Design review of the part built by this model. Coordinates are the model's own, in mm. Coordinates: 2 decimals unless noted, no trailing zeros. Loops run counter-clockwise (first coordinate to the right, second up) from the corner with the lowest first, then second, coordinate; pieces in that order, holes last. Notation, with made-up numbers: (56.25, 19.25) - (72.25, 19.25) arc R10 cw to (72.25, 36.25) - close; hole circle Ø9 at (-33, 53). An arc over 180 degrees is marked (long way). One line per question, with ' | ' between items.
from build123d import *

# Parameters (mm, degrees)
SKETCH1_W           = 10
SKETCH1_H           = 5
BOSS_EXTRUDE1_DEPTH = 0.6
SKETCH2_W           = 1.15
SKETCH2_H           = 2.7
CUT_EXTRUDE1_DEPTH  = 6.622277119
SKETCH3_R           = 0.15
CUT_EXTRUDE2_DEPTH  = 6.622277119


with BuildPart() as part:
    # Sketch1 → Boss-Extrude1 (new body)
    with BuildSketch(Plane.XY):
        Rectangle(SKETCH1_W, SKETCH1_H)
    extrude(amount=BOSS_EXTRUDE1_DEPTH)

    # Sketch2 → Cut-Extrude1 (cut, through all)
    with BuildSketch(Plane.XY.offset(0.6)):
        with Locations((-4.425, -1.15)):
            Rectangle(SKETCH2_W, SKETCH2_H)
    extrude(amount=-CUT_EXTRUDE1_DEPTH, mode=Mode.SUBTRACT)

    # Sketch3 → Cut-Extrude2 (cut, through all)
    with BuildSketch(Plane.XY.offset(0.6)):
        with Locations((-4.4, 1.85)):
            Circle(SKETCH3_R)
        with Locations((-4.4, 1.35)):
            Circle(SKETCH3_R)
        with Locations((-4.4, 0.85)):
            Circle(SKETCH3_R)
    extrude(amount=-CUT_EXTRUDE2_DEPTH, mode=Mode.SUBTRACT)


solid = part.part
Q1. Take a section at D-D (y = -0.3). Give the boundary of the cut face in (x, z), plus the area to 3 significant figures.
Returned:
outline: (-3.85, 0) - (5, 0) - (5, 0.6) - (-3.85, 0.6) - close | area: 5.31 mm²
Q2. To check wall thickness, follow line 1 along Y through (x, z) = (-4.4, 0.45); line 2 along Y through (x, z) = (-4, 0.25); line 3 along X through (y, z) = (-1.65, 0.2). State the ranges of each line that lie inside material, in increasing order.
Returned:
line 1: y = 0.2 to 0.7, 1 to 1.2, 1.5 to 1.7, 2 to 2.5 | line 2: y = 0.2 to 2.5 | line 3: x = -3.85 to 5
Q3. Take a section at A-A (x = -4.4). Give the boundary of the cut face in (y, z).
Returned:
outline: (0.2, 0) - (0.7, 0) - (0.7, 0.6) - (0.2, 0.6) - close; (1, 0) - (1.2, 0) - (1.2, 0.6) - (1, 0.6) - close; (1.5, 0) - (1.7, 0) - (1.7, 0.6) - (1.5, 0.6) - close; (2, 0) - (2.5, 0) - (2.5, 0.6) - (2, 0.6) - close
Q4. Take a section at B-B (y = 0.85). Give the boundary of the cut face in (x, z), plus the area to 3 significant figures.
Returned:
outline: (-5, 0) - (-4.55, 0) - (-4.55, 0.6) - (-5, 0.6) - close; (-4.25, 0) - (5, 0) - (5, 0.6) - (-4.25, 0.6) - close | area: 5.82 mm²
Q5. Take a section at C-C (z = 0.25). Give the boundary of the cut face in (x, y).
Returned:
outline: (-5, 0.2) - (-3.85, 0.2) - (-3.85, -2.5) - (5, -2.5) - (5, 2.5) - (-5, 2.5) - close; hole circle Ø0.3 at (-4.4, 0.85); hole circle Ø0.3 at (-4.4, 1.35); hole circle Ø0.3 at (-4.4, 1.85)
